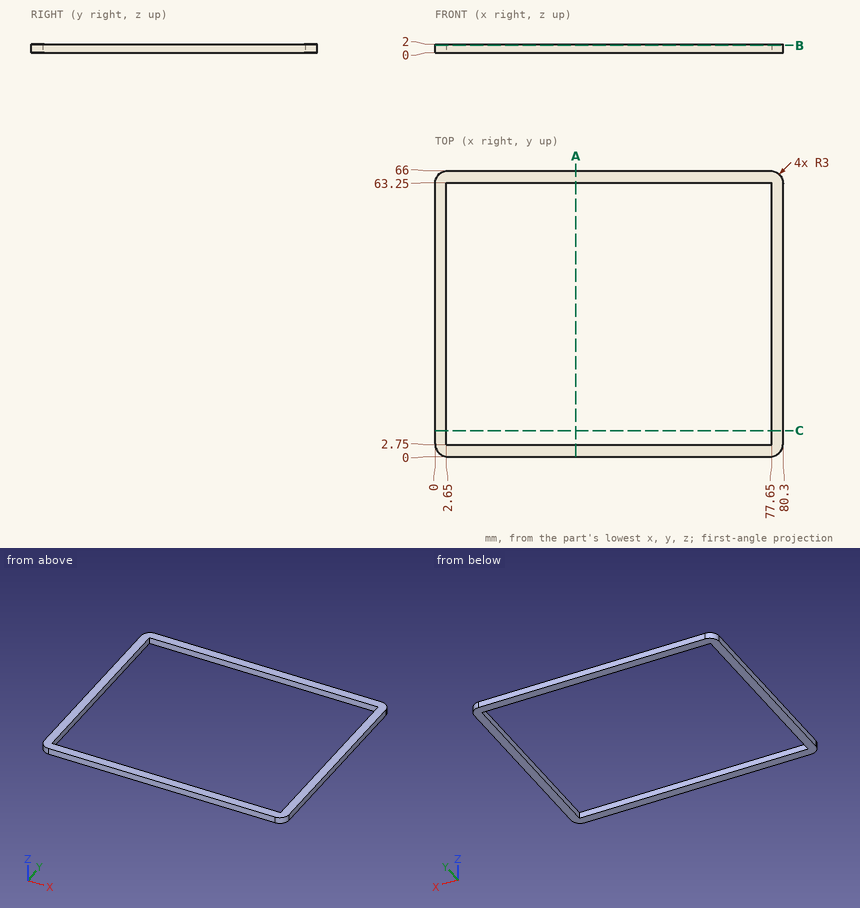
Part print with two shaded views. Sizes in mm from the minimum x, y, z corner. Coordinates: 2 decimals unless noted, no trailing zeros. Write each loop counter-clockwise with the first axis right and the second up, starting at its lowest first coordinate (ties: lowest second). Pieces come first, ordered by that corner, then holes. Notation, with made-up numbers: (89.25, -11.5) -> (135.25, -11.5) arc R4 ccw to (135.25, -5.5) -> close; hole circle Ø8 at (6, -13.5). An arc over 180 degrees is marked (long way). Return JSON: item names as keys, results as strings. Group by question number.
Q1. Cut at C-C, the plane y = 6. Give the cut face in (x, z).
Q2. Drill centre lines: line 1 (Y direction, x = 12, z = 1.75); line 2 (X direction, y = 62, z = 1.2). Where is each one in solid material? Low to high.
Q3. Cut at A-A, the plane x = 32.5. Give the cut face in (y, z).
Q4. Cut at B-B, the plane z = 1.7. Give the cut face in (x, y), then the cut area to 3 significant figures.
Returned:
{
 "1": {"outline": "(0, 0) -> (2.65, 0) -> (2.65, 2) -> (0, 2) -> close; (77.65, 0) -> (80.3, 0) -> (80.3, 2) -> (77.65, 2) -> close"},
 "2": {"line 1": "y = 0 to 2.75, 63.25 to 66", "line 2": "x = 0 to 2.65, 77.65 to 80.3"},
 "3": {"outline": "(0, 0) -> (2.75, 0) -> (2.75, 2) -> (0, 2) -> close; (63.25, 0) -> (66, 0) -> (66, 2) -> (63.25, 2) -> close"},
 "4": {"outline": "(0, 3) arc R3 ccw to (3, 0) -> (77.3, 0) arc R3 ccw to (80.3, 3) -> (80.3, 63) arc R3 ccw to (77.3, 66) -> (3, 66) arc R3 ccw to (0, 63) -> close; hole (2.65, 2.75) -> (77.65, 2.75) -> (77.65, 63.25) -> (2.65, 63.25) -> close", "area": "755 mm2"}
}
